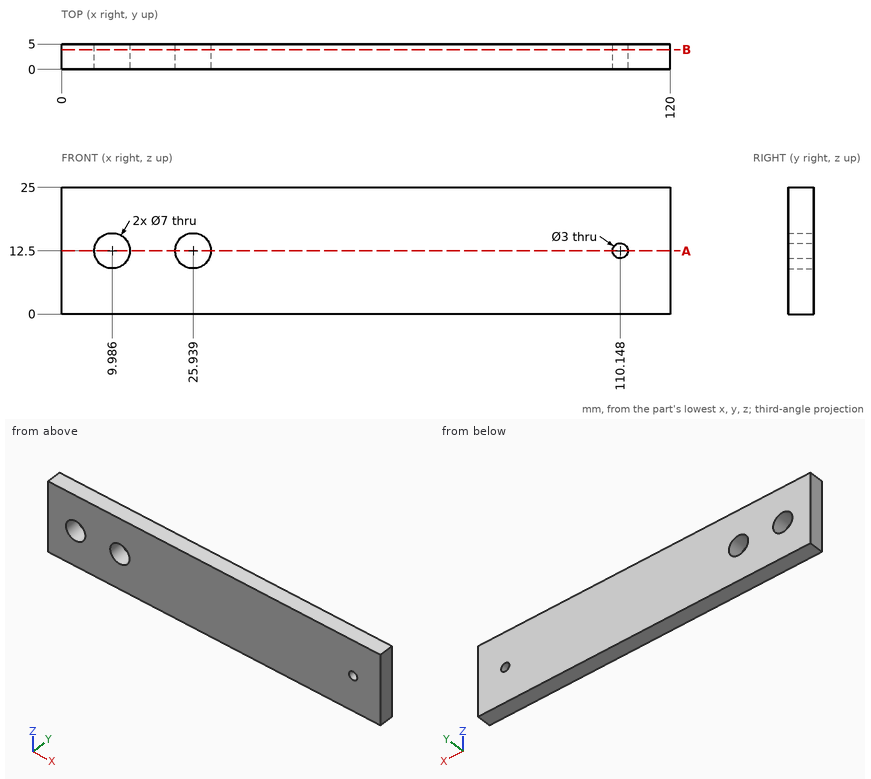
Answer from the drawing. Dimensions are ordinates in mm from the lowest x, y and z of the part. Give positions to 0.01 mm unless a question says otherwise; leave off trailing zeros. Loops run counter-clockwise (first coordinate to the right, second up) from the corner with the lowest first, then second, coordinate; pieces in that order, holes last. Notation, with made-up numbers: (-24.75, 74.5) -> (-6.75, 74.5) arc R31 ccw to (-6.75, 112.5) -> close; hole circle Ø10 at (-13, 34.25). An arc over 180 degrees is marked (long way). Use a Markdown table: item, result.
Q1. Section A-A, the plane z = 12.5 is taken. Determine the outline of the cut face in (x, y) (1 decimal), then the cut area to 3 significant figures.
Solved:
| item | result |
|---|---|
| outline | (0, 0) -> (6.5, 0) -> (6.5, 5) -> (0, 5) -> close; (13.5, 0) -> (22.4, 0) -> (22.4, 5) -> (13.5, 5) -> close; (29.4, 0) -> (108.6, 0) -> (108.6, 5) -> (29.4, 5) -> close; (111.6, 0) -> (120, 0) -> (120, 5) -> (111.6, 5) -> close |
| area | 515 mm^2 |
Q2. Section B-B, the plane y = 3.9 is taken. Determine the outline of the cut face in (x, z) (1 decimal).
Solved:
| item | result |
|---|---|
| outline | (0, 0) -> (120, 0) -> (120, 25) -> (0, 25) -> close; hole circle Ø7 at (10, 12.5); hole circle Ø7 at (25.9, 12.5); hole circle Ø3 at (110.1, 12.5) |
Q3. Find the intervals of material crossed by line 1 along X through (y, z) = (2.35, 12.5) (1 decimal); line 2 along X through (y, z) = (2.3, 15) (1 decimal), in increasing order.
Solved:
| item | result |
|---|---|
| line 1 | x = 0 to 6.5, 13.5 to 22.4, 29.4 to 108.6, 111.6 to 120 |
| line 2 | x = 0 to 7.5, 12.4 to 23.5, 28.4 to 120 |
